Autodesk Inventor part; units mm, degrees
ref_plane "YZ Plane" through (0, 0, 0) normal (1, 0, 0) x (0, 1, 0)
ref_plane "XZ Plane" through (0, 0, 0) normal (0, 1, 0) x (-1, 0, 0)
ref_plane "XY Plane" through (0, 0, 0) normal (0, 0, 1) x (1, 0, 0)
sketch "Skizze1" plane through (0, 0, 0) normal (0, 0, 1) x (1, 0, 0)
  line L0 (-24, 0) -> (144, 0)
  line L1 (0, -32) -> (0, 192)
  line L2 (0, 0) -> (120, 0)
  line L3 (120, 0) -> (120, 160)
  line L4 (120, 160) -> (0, 160)
  line L5 (0, 160) -> (0, 0)
  point P0 (0, 160)
  dimension "d0" = 120
  dimension "d1" = 160
extrude "Extrusion1" add sketch "Skizze1" along normal blind 140
sketch "Skizze2" plane through (0, 0, 0) normal (0, 0, -1) x (-1, 0, 0)
  line L0 (-10, 10) -> (-110, 10)
  line L1 (-110, 10) -> (-110, 40)
  line L2 (-110, 40) -> (-10, 40)
  line L3 (-10, 40) -> (-10, 10)
  line L4 (0, 0) -> (-120, 0)
  line L5 (0, 160) -> (0, 0)
  line L6 (-120, 0) -> (-120, 160)
  dimension "d4" = 10
  dimension "d5" = 10
  dimension "d6" = 10
  dimension "d7" = 30
extrude "Extrusion2" cut sketch "Skizze2" against normal blind 130
sketch "Skizze3" plane through (0, 160, 0) normal (0, 1, 0) x (1, 0, 0)
  line L0 (110, -130) -> (10, -130)
  line L1 (10, -130) -> (10, -10)
  line L2 (10, -10) -> (110, -10)
  line L3 (110, -10) -> (110, -130)
  line L4 (120, -140) -> (0, -140)
  line L5 (0, 0) -> (0, -140)
  line L6 (120, 0) -> (120, -140)
  line L7 (120, 0) -> (0, 0)
  dimension "d10" = 10
  dimension "d11" = 10
  dimension "d12" = 10
  dimension "d13" = 10
extrude "Extrusion3" cut sketch "Skizze3" against normal blind 130 contours L0 L1 L2 L3
properties part number "EierkocherTeil2" material "Acetalharz, Schwarz"
Part model, mm, in its own coordinate system. A direction names the side the tool comes from. Round coordinates to 2 decimals unless told otherwise and drop trailing zeros. Write each loop counter-clockwise with the first axis right and the second up, starting at its lowest first coordinate (ties: lowest second). Pieces come first, ordered by that corner, then holes. Notation, with made-up numbers: M 41.25,11 L 52.25,11 A12 ccw 52.25,24 Z; hole C -34.75,78.25 d6. An arc over 180 degrees is marked long. Return JSON: item names as keys, results as strings. Group by question number.
(1) Saw through at A-A on x = 15. Write the cut outline in (y, z), then the cut area to 3 significant figures.
(2) Pin check, flat tip, straight feed: pin 1 Ø1 at (x, z) = (67, 20) entering from +Y. Stop position of the tip, or through.
(3) Saw through at B-B on y = 47. Write the cut outline in (x, z).
(4) Two-plate mould, pull along X, no slides. Class faces 4 (the face through (120, 79, 69)), 5 (the face through (59, 0, 69)), 6 (the face through (10, 86, 66)): +X half, -X half, draft (parallel to the pull), parting line (faces both ways), or undercut.
(5) Drill centre lines: probe 1 along X at (y, z) = (45, 72.5); probe 2 along Z at (x, y) = (71, 74.5); probe 3 along Y at (x, z) = (94.5, 6.5). Where is each one in solid material? Low to high.
(6) Saw through at C-C on z = 44.5. Write the cut outline in (x, y), then the cut area to 3 significant figures.
(7) Saw through at D-D on y = 30. Write the cut outline in (x, z), then the cut area to 3 significant figures.
(8) Which spindle directions (+Z, -Z, +X, -X, +Y, -Y) get a long thin tool onto all of the face, cutting with end or side? Do faces 1 (the face through (59, 81, 140)), 2 (the face through (59, 101, 10)), 3 (the face through (61, 40, 5)). Say none if no direction does.
Returned:
{
 "1": {"outline": "M 0,0 L 10,0 L 10,130 L 160,130 L 160,140 L 0,140 Z; M 40,0 L 160,0 L 160,10 L 40,10 Z", "area": "4,100 mm²"},
 "2": {"pin 1": "y = 10"},
 "3": {"outline": "M 0,0 L 120,0 L 120,140 L 0,140 Z; hole M 10,10 L 110,10 L 110,130 L 10,130 Z"},
 "4": {"face 4": "+X half", "face 5": "draft", "face 6": "undercut"},
 "5": {"probe 1": "0 to 10, 110 to 120", "probe 2": "0 to 10, 130 to 140", "probe 3": "0 to 10, 40 to 160"},
 "6": {"outline": "M 0,0 L 120,0 L 120,160 L 110,160 L 110,10 L 10,10 L 10,160 L 0,160 Z", "area": "4,200 mm²"},
 "7": {"outline": "M 0,0 L 10,0 L 10,130 L 110,130 L 110,0 L 120,0 L 120,140 L 0,140 Z", "area": "3,800 mm²"},
 "8": {"face 1": "+Z, +X, -X, +Y, -Y", "face 2": "+Y", "face 3": "-Z"}
}
